from build123d import *

# Parameters (mm, degrees)
SKETCH1_R           = 2.22670754
SKETCH1_R_2         = 2.7559
BOSS_EXTRUDE1_DEPTH = 6.35
SKETCH2_R           = 3.175
BOSS_EXTRUDE2_DEPTH = 12.7
BOSS_EXTRUDE3_DEPTH = 2.54
FILLET1_R           = 2.54


with BuildPart() as part:
    # Sketch1 → Boss-Extrude1 (new body)
    with BuildSketch(Plane(origin=(0, 0, 0), x_dir=(0, 0, -1), z_dir=(1, 0, 0))):
        with BuildLine():
            Line((-44.45, 12.7), (-44.45, -12.7))
            Line((-44.45, -12.7), (-1.778, -25.146))
            ThreePointArc((-1.778, -25.146), (3.81, -24.13), (6.35, -19.05))
            Line((6.35, -19.05), (6.35, 19.05))
            ThreePointArc((6.35, 19.05), (3.81, 24.13), (-1.778, 25.146))
            Line((-1.778, 25.146), (-44.45, 12.7))
        make_face()
        with Locations((-38.1, 0)):
            Circle(SKETCH1_R, mode=Mode.SUBTRACT)
        with Locations((-9.652, 0)):
            Circle(SKETCH1_R, mode=Mode.SUBTRACT)
        with Locations((0, -19.05)):
            Circle(SKETCH1_R_2, mode=Mode.SUBTRACT)
        with Locations((0, 19.05)):
            Circle(SKETCH1_R_2, mode=Mode.SUBTRACT)
    extrude(amount=-BOSS_EXTRUDE1_DEPTH)

    # Sketch2 → Boss-Extrude2 (add)
    with BuildSketch(Plane(origin=(0, 0, 0), x_dir=(0, 0, -1), z_dir=(1, 0, 0))):
        with Locations((0, -4.7625)):
            Circle(SKETCH2_R)
        with Locations((0, 4.7625)):
            Circle(SKETCH2_R)
    extrude(amount=BOSS_EXTRUDE2_DEPTH)

    # Sketch4 → Boss-Extrude3 (add)
    with BuildSketch(Plane(origin=(12.7, 0, 0), x_dir=(0, 0, -1), z_dir=(1, 0, 0))):
        with BuildLine():
            Line((-3.175, 4.7625), (-3.175, -4.7625))
            ThreePointArc((-3.175, -4.7625), (-2.600807741, -6.583605185), (-1.085913955, -7.746024071))
            Line((-1.085913955, -7.746024071), (4.760575332, -9.873972147))
            ThreePointArc((4.760575332, -9.873972147), (6.404796784, -7.549757281), (6.985, -4.7625))
            Line((6.985, -4.7625), (6.985, 4.7625))
            ThreePointArc((6.985, 4.7625), (6.404796784, 7.549757281), (4.760575332, 9.873972147))
            Line((4.760575332, 9.873972147), (-1.085913955, 7.746024071))
            ThreePointArc((-1.085913955, 7.746024071), (-2.600807741, 6.583605185), (-3.175, 4.7625))
        make_face()
    extrude(amount=BOSS_EXTRUDE3_DEPTH)

    # Fillet1
    fillet1_edges = [part.edges().sort_by_distance(p)[0] for p in [
        (-3.175, -12.7, 44.45),
        (-3.175, 12.7, 44.45),
        (13.97, -9.873972147, -4.760575332),
        (13.97, 9.873972147, -4.760575332),
    ]]
    fillet(fillet1_edges, radius=FILLET1_R)


solid = part.part
Part model, mm, in its own coordinate system. A direction names the side the tool comes from. Coordinates: 2 decimals unless noted, no trailing zeros. Loops run counter-clockwise (first coordinate to the right, second up) from the corner with the lowest first, then second, coordinate; pieces in that order, holes last. Notation, with made-up numbers: (0.5, 38) -> (49.5, 38) arc R27 ccw to (49.5, 69) -> close; hole circle Ø4 at (-9.75, 21.5). An arc over 180 degrees is marked (long way). Use a Markdown table: item, result. Add a question column.
Item 1: Band-saw the part on B-B on x = -4. Write the cut outline in (y, z) (3 decimals), plus the area to 3 significant figures.
Item 2: Pull direction X, two halves, no side cores. Call faces 5 (the flat face through (15.24, 0, -2)), 6 (the flat face through (-3, 0, 44.45)), 7 (the flat face through (-6.35, 0, 14)), 8 (the flat face through (12.7, 0, -3)): +X half, -X half, draft (parallel to the pull), parting line (faces both ways), or undercut.
Item 3: Band-saw the part on C-C on z = 0. Write the cut outline in (x, y).
Item 4: Which spindle directions (+Z, -Z, +X, -X, +Y, -Y) get a long thin tool onto all of the face, cutting with end or side? Do faces 1 (the flat face through (14, 0, 3.175)), 2 (the cylindrical face through (13.988, -9.246, -4.799)), 3 (the flat face through (13.95, 8.51, -1.01)), 4 (the flat face through (-3, 0, -6.35)). Say none if no direction does.
Item 5: Probe probe 1 along Y at (x, z) = (-2, 0); probe 2 along X at (y, z) = (-6, 16.5); probe 3 along Z at (x, y) = (12.25, 5). List the from-to ranges inside material, lowest first.
Item 6: Flat gauge pins, fed straight in: P1, Ø3, axis at x = -2.5, y = -8, coming from the -Z side; P2, Ø6, axis at x = 11, y = -9.5, coming from the -Z side; P3, Ø15, axis at y = -1.5, z = 14.5, coming from the +X side. Where does each tip first touch, or does it go through?
Item 7: Band-saw the part on A-A on y = 0. Write the cut outline in (x, z) (3 decimals), plus the area to 3 significant figures.
Geometry says:
| question | item | result |
|---|---|---|
| 1 | outline | (-25.146, 1.778) arc R6.35 ccw to (-19.05, -6.35) -> (19.05, -6.35) arc R6.35 ccw to (25.146, 1.778) -> (13.233, 42.621) arc R2.54 ccw to (10.795, 44.45) -> (-10.795, 44.45) arc R2.54 ccw to (-13.233, 42.621) -> close; hole circle Ø5.512 at (-19.05, 0); hole circle Ø4.453 at (0, 9.652); hole circle Ø4.453 at (0, 38.1); hole circle Ø5.512 at (19.05, 0) |
| 1 | area | 1,930 mm² |
| 2 | face 5 | +X half |
| 2 | face 6 | draft |
| 2 | face 7 | -X half |
| 2 | face 8 | undercut |
| 3 | outline | (-6.35, -25.4) -> (0, -25.4) -> (0, -21.81) -> (-6.35, -21.81) -> close; (-6.35, -16.29) -> (0, -16.29) -> (0, -7.94) -> (12.7, -7.94) -> (12.7, -8.14) -> (15.24, -8.14) -> (15.24, 8.14) -> (12.7, 8.14) -> (12.7, 7.94) -> (0, 7.94) -> (0, 16.29) -> (-6.35, 16.29) -> close; (-6.35, 21.81) -> (0, 21.81) -> (0, 25.4) -> (-6.35, 25.4) -> close; hole (0, -1.59) -> (12.7, -1.59) -> (12.7, 1.59) -> (0, 1.59) -> close |
| 4 | face 1 | +Z, +X, +Y, -Y |
| 4 | face 2 | +X, -Y |
| 4 | face 3 | +Z, +X, +Y |
| 4 | face 4 | -Z, -X, +Y, -Y |
| 5 | probe 1 | -25.4 to -21.81, -16.29 to 16.29, 21.81 to 25.4 |
| 5 | probe 2 | -6.35 to 0 |
| 5 | probe 3 | -3.17 to 3.17 |
| 6 | P1 | z = -6.35 |
| 6 | P2 | z = -6.61 |
| 6 | P3 | x = 0 |
| 7 | outline | (-6.35, -6.35) -> (0, -6.35) -> (0, 7.425) -> (-6.35, 7.425) -> close; (-6.35, 11.879) -> (0, 11.879) -> (0, 35.873) -> (-6.35, 35.873) -> close; (-6.35, 40.327) -> (0, 40.327) -> (0, 44.45) -> (-6.35, 44.45) -> close; (12.7, -6.985) -> (15.24, -6.985) -> (15.24, 3.175) -> (12.7, 3.175) -> close |
| 7 | area | 292 mm² |
